Print and shaded views of the part. All mm, measured from the part's lowest x, y and z. A direction names the side the tool comes from. Give positions to 0.01 mm unless a question says otherwise; leave off trailing zeros. Order: outer loops, then holes, each group sorted by start corner. A loop starts at its lowest first (then second) coordinate and runs counter-clockwise, first axis right, second up. Notation, with made-up numbers: (-21.75, 44.5) -> (12.25, 44.5) arc R34 cw to (12.25, 82.5) -> close; hole circle Ø11 at (41, -35). An arc over 180 degrees is marked (long way). One line per question, with ' | ' between items. Start each with the question number.
(1) Drill centre lines: L1, parallel to Z at x = 15, y = 5; L2, parallel to Y at x = 11.75, z = 41.5; L3, parallel to X at y = 8, z = 9. Where is each one in solid material? Low to high. Write a range as from..to.
(2) Cut at A-A (x = 15). Give the cut face in (y, z), then the cut area to 3 significant figures.
(3) Cut at D-D (y = 6). Give the cut face in (x, z), then the cut area to 3 significant figures.
(4) Pin check, flat tips, straight feed: pin 1 Ø1.5 at (x, y) = (6, 35) entering from +Z; pin 2 Ø8 at (x, z) = (12.5, 66.5) entering from +Y; pin 3 Ø5 at (x, z) = (14.5, 10) entering from +Y. Stop position of each tip, or through.
(5) Pull direction Y, two halves, no side cores. Call the marked faces 1, 2, 3 and 4: +Y half, -Y half, draft (parallel to the pull), parting line (faces both ways), or undercut.
(6) Which spindle directions (+Z, -Z, +X, -X, +Y, -Y) get a long thin tool onto all of the face, cutting with end or side? Do the marked faces 5, 6 and 7. Say none if no direction does.
(7) Cut at B-B (z = 41.5). Give the cut face in (x, y), then the cut area to 3 significant figures.
(8) Cut at C-C (y = 40). Give the cut face in (x, z), then the cut area to 3 significant figures.
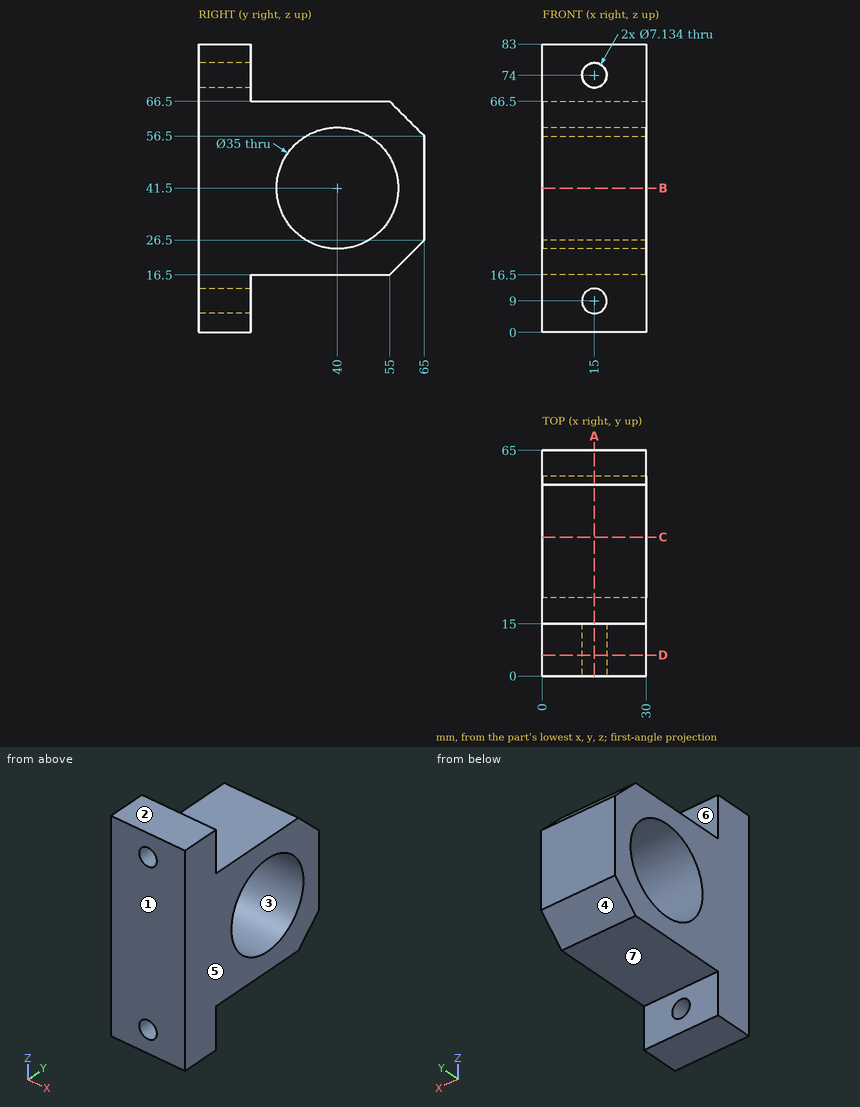
Result set:
1) L1: z = 0..5.43, 12.57..70.43, 77.57..83 | L2: y = 0..22.5, 57.5..65 | L3: x = 0..11.43, 18.57..30
2) outline: (0, 0) -> (15, 0) -> (15, 5.43) -> (0, 5.43) -> close; (0, 12.57) -> (15, 12.57) -> (15, 16.5) -> (55, 16.5) -> (65, 26.5) -> (65, 56.5) -> (55, 66.5) -> (15, 66.5) -> (15, 70.43) -> (0, 70.43) -> close; (0, 77.57) -> (15, 77.57) -> (15, 83) -> (0, 83) -> close; hole circle Ø35 at (40, 41.5) | area: 2,470 mm2
3) outline: (0, 0) -> (30, 0) -> (30, 83) -> (0, 83) -> close; hole circle Ø7.13 at (15, 9); hole circle Ø7.13 at (15, 74) | area: 2,410 mm2
4) pin 1: stops at z = 66.5 | pin 2: stops at y = 59 | pin 3: stops at y = 15
5) face 1: -Y half | face 2: draft | face 3: undercut | face 4: +Y half
6) face 5: +Z, -Z, +X, +Y, -Y | face 6: +Z, +X, -X, +Y | face 7: -Z, +X, -X, +Y
7) outline: (0, 0) -> (30, 0) -> (30, 22.5) -> (0, 22.5) -> close; (0, 57.5) -> (30, 57.5) -> (30, 65) -> (0, 65) -> close | area: 900 mm2
8) outline: (0, 16.5) -> (30, 16.5) -> (30, 24) -> (0, 24) -> close; (0, 59) -> (30, 59) -> (30, 66.5) -> (0, 66.5) -> close | area: 450 mm2
